Part model, mm, in its own coordinate system. A direction names the side the tool comes from. Round coordinates to 2 decimals unless told otherwise and drop trailing zeros. Loops run counter-clockwise (first coordinate to the right, second up) from the corner with the lowest first, then second, coordinate; pieces in that order, holes last. Notation, with made-up numbers: (24.25, 47) -> (66.25, 47) arc R27 ccw to (66.25, 74) -> close; hole circle Ø11 at (-11, 65.25). An arc over 180 degrees is marked (long way). Answer as CSV lines item,"result".
from build123d import *

# Parameters (mm, degrees)
SKETCH1_R           = 16
SKETCH1_R_2         = 6.25
BOSS_EXTRUDE1_DEPTH = 100
SKETCH2_W           = 40
SKETCH2_H           = 55
CUT_EXTRUDE1_DEPTH  = 20
SKETCH3_W           = 56
SKETCH3_H           = 46
BOSS_EXTRUDE2_DEPTH = 28
SKETCH4_R           = 8
BOSS_EXTRUDE3_DEPTH = 26


with BuildPart() as part:
    # Sketch1 → Boss-Extrude1 (new body)
    with BuildSketch(Plane(origin=(0, 0, 0), x_dir=(1, 0, 0), z_dir=(0, 1, 0))):
        with Locations(Location((0, 0, 0), (0, 0, 270))):
            Circle(SKETCH1_R)
        with Locations(Location((0, 0, 0), (0, 0, 270))):
            Circle(SKETCH1_R_2, mode=Mode.SUBTRACT)
    extrude(amount=BOSS_EXTRUDE1_DEPTH)

    # Sketch2 → Cut-Extrude1 (cut, symmetric)
    with BuildSketch(Plane.XY):
        with Locations((0, 25.5)):
            Rectangle(SKETCH2_W, SKETCH2_H)
    extrude(amount=CUT_EXTRUDE1_DEPTH, both=True, mode=Mode.SUBTRACT)

    # Sketch3 → Boss-Extrude2 (add, symmetric)
    with BuildSketch(Plane.XY):
        with Locations((0, 77)):
            Rectangle(SKETCH3_W, SKETCH3_H)
    extrude(amount=BOSS_EXTRUDE2_DEPTH, both=True)

    # Sketch4 → Boss-Extrude3 (add, symmetric)
    with BuildSketch(Plane.XY):
        with Locations((0, 76)):
            Circle(SKETCH4_R)
    extrude(amount=BOSS_EXTRUDE3_DEPTH, both=True)


solid = part.part
Q1. Saw through at B-B, the plane x = -24. Write the cut outline in (y, z), then the cut area to 3 significant figures.
Geometry results:
outline,"(54, -28) -> (100, -28) -> (100, 28) -> (54, 28) -> close"
area,"2,580 mm2"
Q2. Two-plate mould, pull along Z, no slides. Class faces 3 (the face through (28, 77, 0)), 4 (the face through (0, 77, -28)), 5 (the face through (0, 54, 0)), 6 (the face through (1.88, 53.49, 5.96)): pulls with the +Z half, pulls with the -Z half, needs draft (parallel to the pull), parting line crosses it, or undercut.
Geometry results:
face 3,"needs draft"
face 4,"pulls with the -Z half"
face 5,"undercut"
face 6,"undercut"
Q3. Drop a flat-ended pin along its axis: P1, Ø4, axis at x = -2, z = 0.5, coming from the -Y side. Give the stop position or say it passes through.
Geometry results:
P1,"y = 54"
Q4. Drill centre lines: line 1 along Z through (x, y) = (0, 53.55); line 2 along Y through (x, z) = (7.5, -23.5). Where is each one in solid material? Low to high.
Geometry results:
line 1,"-16 to -6.25, 6.25 to 16"
line 2,"54 to 100"
Q5. Saw through at A-A, the plane z = -19. Write the cut outline in (x, y).
Geometry results:
outline,"(-28, 54) -> (28, 54) -> (28, 100) -> (-28, 100) -> close"
Q6. Which spindle directions (+Z, -Z, +X, -X, +Y, -Y) get a long thin tool onto all of the face, cutting with end or side? Do faces 1 (the face through (-13, 54, -12)), 2 (the face through (0, 77, 28)). Say none if no direction does.
Geometry results:
face 1,"-Y"
face 2,"+Z, +X, -X, +Y, -Y"
